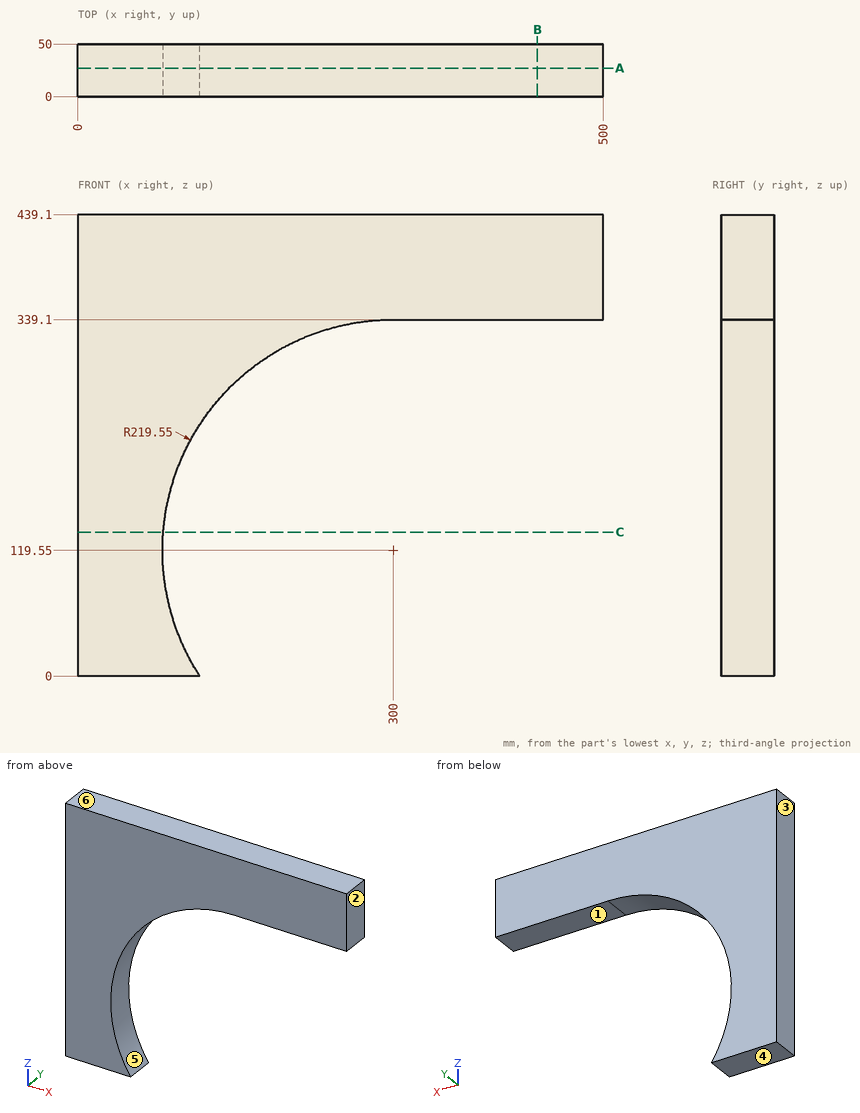
The figure shows three views and two pictorial views of one solid part (mm, origin at its lowest corner). Answer the questions. A direction names the side the tool comes from. Round coordinates to 2 decimals unless told otherwise and drop trailing zeros. Order: outer loops, then holes, each group sorted by start corner. A loop starts at its lowest first (then second) coordinate and runs counter-clockwise, first axis right, second up. Notation, with made-up numbers: M -28.5,-5.5 L -17.5,-5.5 A14 cw -17.5,10.5 Z; hole C 12.25,-24.5 d10. An arc over 180 degrees is marked long. Answer in a Markdown table with one row per item. Add a question column.
1) The part is cut by section A-A on y = 27. Determine the outline of the cut face in (x, z), plus the area to 3 significant figures.
2) Determine the mould class of the marked faces 3, 4, 5 and 6 for opening direction Z: pulls with the +Z half, pulls with the -Z half, needs draft (parallel to the pull), parting line crosses it, or undercut.
3) Which of the six approach directions +Z, -Z, +X, -X, +Y, -Y give full straight-line access (tool end or side, diameter ignored) to the marked faces 1 and 2?
4) The part is cut by section B-B on x = 437. Determine the outline of the cut face in (y, z).
5) Flat-ended cylindrical pins translate along their axes: pin 1 Ø1.5 at (y, z) = (27, 135) entering from +X; pin 2 Ø25 at (x, y) = (372, 35) entering from -Z; pin 3 Ø1.5 at (x, y) = (163.5, 38.5) entering from -Z. Find the tip coordinate at first contact, or state that the pin passes through.
6) The part is cut by section C-C on z = 137. Determine the outline of the cut face in (x, y).
7) Consider line 1 along Z through (x, y) = (331, 27); line 2 along X through (y, z) = (31, 60.5); line 3 along Z through (x, y) = (105.5, 31). Determine where each line is inside the solid, lowest interval first. Write a range as from..to.
Findings below:
| question | item | result |
|---|---|---|
| 1 | outline | M 0,0 L 115.85,0 A219.55 cw 300,339.1 L 500,339.1 L 500,439.1 L 0,439.1 Z |
| 1 | area | 89,000 mm² |
| 2 | face 3 | needs draft |
| 2 | face 4 | pulls with the -Z half |
| 2 | face 5 | undercut |
| 2 | face 6 | pulls with the +Z half |
| 3 | face 1 | -Z, +X, +Y, -Y |
| 3 | face 2 | +Z, -Z, +X, +Y, -Y |
| 4 | outline | M 0,339.1 L 50,339.1 L 50,439.1 L 0,439.1 Z |
| 5 | pin 1 | stops at x = 81.05 |
| 5 | pin 2 | stops at z = 339.1 |
| 5 | pin 3 | stops at z = 290.91 |
| 6 | outline | M 0,0 L 81.14,0 L 81.14,50 L 0,50 Z |
| 7 | line 1 | z = 339.1..439.1 |
| 7 | line 2 | x = 0..88.54 |
| 7 | line 3 | z = 0..17.71, 221.39..439.1 |
